Read the model definition and answer for the solid it produces. Units are mm, in the model's axes. Coordinates: 2 decimals unless noted, no trailing zeros. Order: outer loops, then holes, each group sorted by start corner. A loop starts at its lowest first (then second) coordinate and runs counter-clockwise, first axis right, second up. Notation, with made-up numbers: (11.25, -0.75) -> (52.25, -0.75) arc R20 ccw to (52.25, 36.25) -> close; hole circle Ø9 at (2.25, 77). An arc over 180 degrees is marked (long way). Answer as a JSON object with one key per item and string values. Group by question number.
1) Given pin 1 (1 mm diameter, centred on y = 2.5, z = -41, fed in from +X); pin 2 (2 mm diameter, centred on y = 2, z = -181.5, fed in from -X); pin 3 (2.5 mm diameter, centred on y = 4.5, z = -283.5, fed in from +X); pin 4 (2.5 mm diameter, centred on x = -286, y = 2, fed in from +Z), each flat-ended and moving along its own axis, determine where each tip first touches the part or whether it passes through.
2) Section B-B on z = -165.5 is taken. Determine the outline of the cut face in (x, y), and give its area (3 significant figures).
3) Section A-A on y = 4.5 is taken. Determine the outline of the cut face in (x, z), and give its area (3 significant figures).
4) Consider L1, parallel to Z at x = -110, y = 5.5; L2, parallel to Z at x = -104, y = 1.25; L3, parallel to X at y = 1.5, z = -249.5. Determine where each line is inside the solid, lowest interval first.
from build123d import *

# Parameters (mm, degrees)
BOSS_EXTRUDE2_DEPTH = 6.35


with BuildPart() as part:
    # Sketch1 → Boss-Extrude2 (new body)
    with BuildSketch(Plane(origin=(0, 0, 0), x_dir=(1, 0, 0), z_dir=(0, 1, 0))):
        with BuildLine():
            Line((0, 288.036), (0, 291.211))
            ThreePointArc((0, 291.211), (-56.812447765, 285.615462292), (-111.441625022, 269.043882542))
            Line((-111.441625022, 269.043882542), (-109.011585227, 263.177247511))
            ThreePointArc((-109.011585227, 263.177247511), (-55.57362422, 279.387475761), (0, 284.861))
            Line((0, 284.861), (6.35, 284.861))
            Line((6.35, 284.861), (6.35, 288.036))
            Line((6.35, 288.036), (0, 288.036))
        make_face()
        with BuildLine():
            ThreePointArc((0, 284.861), (-55.57362422, 279.387475761), (-109.011585227, 263.177247511))
            ThreePointArc((-109.011585227, 263.177247511), (-201.427144796, 201.427144796), (-263.177247511, 109.011585227))
            ThreePointArc((-263.177247511, 109.011585227), (-279.387475761, 55.57362422), (-284.861, 0))
            Line((-284.861, 0), (-281.686, 0))
            ThreePointArc((-281.686, 0), (-199.182080765, 199.182080765), (0, 281.686))
            Line((0, 281.686), (0, 284.861))
        make_face()
        with BuildLine():
            Line((-263.177247511, 109.011585227), (-269.043882542, 111.441625022))
            ThreePointArc((-269.043882542, 111.441625022), (-285.615462292, 56.812447765), (-291.211, 0))
            Line((-291.211, 0), (-288.036, 0))
            Line((-288.036, 0), (-288.036, 6.35))
            Line((-288.036, 6.35), (-284.861, 6.35))
            Line((-284.861, 6.35), (-284.861, 0))
            ThreePointArc((-284.861, 0), (-279.387475761, 55.57362422), (-263.177247511, 109.011585227))
        make_face()
    extrude(amount=BOSS_EXTRUDE2_DEPTH)


solid = part.part
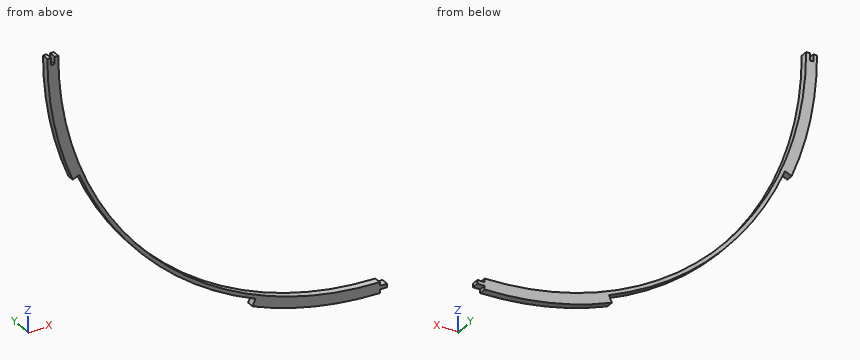
Worked answers:
{
 "1": {"pin 1": "stops at x = -278.61", "pin 2": "stops at x = -220.38", "pin 3": "stops at x = 0", "pin 4": "stops at z = 0"},
 "2": {"outline": "(-231.85, 0) -> (-227.94, 0) -> (-227.94, 6.35) -> (-231.85, 6.35) -> close", "area": "24.8 mm²"},
 "3": {"outline": "(-291.21, 0) arc R291.21 ccw to (-269.04, -111.44) -> (-263.18, -109.01) arc R284.86 ccw to (-109.01, -263.18) -> (-111.44, -269.04) arc R291.21 ccw to (0, -291.21) -> (0, -288.04) -> (6.35, -288.04) -> (6.35, -284.86) -> (0, -284.86) -> (0, -281.69) arc R281.69 cw to (-281.69, 0) -> (-284.86, 0) -> (-284.86, -6.35) -> (-288.04, -6.35) -> (-288.04, 0) -> close", "area": "2,850 mm²"},
 "4": {"L1": "z = -269.64 to -265.56, -262.77 to -259.32", "L2": "z = -272.01 to -261.78", "L3": "x = -137.46 to -130.75"}
}
